from build123d import *

# Parameters (mm, degrees)
F0_W           = 101.6
F0_H           = 50.8
F1_DEPTH       = 101.6
F3_D           = 5.5
F3_CBORE_D     = 9.75
F3_CBORE_DEPTH = 5
F4_R           = 12.7
F5_W           = 38.1
F5_H           = 63.5
F6_DEPTH       = 25.4
F7_R           = 12.7
F8_SIZE        = 6.35


with BuildPart() as f1:
    # F0 (on Top) → F1 (new body, symmetric)
    with BuildSketch(Plane.XY):
        Rectangle(F0_W, F0_H)
    extrude(amount=F1_DEPTH, both=True)

    # F3 (through all)
    with Locations(Plane.XZ.offset(25.4)):
        with Locations((-9.4546508044, 80.2069678903), (23.0063218623, 55.3097166121), (-16.0729084164, -29.151847586), (22.0608543605, -34.1943278909)):
            CounterBoreHole(F3_D / 2, F3_CBORE_D / 2, F3_CBORE_DEPTH)

    # F4
    f4_edges = [f1.edges().sort_by_distance(p)[0] for p in [
        (-50.8, 0, 101.6),
        (50.8, 0, 101.6),
        (-50.8, 0, -101.6),
        (50.8, 0, -101.6),
    ]]
    fillet(f4_edges, radius=F4_R)

    # F5 (on face) → F6 (cut)
    with BuildSketch(Plane.XZ.offset(25.4)):
        with Locations((-19.05, 19.05)):
            Rectangle(F5_W, F5_H)
    extrude(amount=-F6_DEPTH, mode=Mode.SUBTRACT)

    # F7
    f7_edges = [f1.edges().sort_by_distance(p)[0] for p in [
        (0, -12.7, 50.8),
        (-38.1, -12.7, 50.8),
        (-38.1, -12.7, -12.7),
        (0, -12.7, -12.7),
    ]]
    fillet(f7_edges, radius=F7_R)

    # F8
    f8_edges = [f1.edges().sort_by_distance(p)[0] for p in [
        (-34.380256, -25.4, 47.080256),
    ]]
    chamfer(f8_edges, length=F8_SIZE)


solid = f1.part
The model under review builds one solid part; all positions refer to its coordinate system, in mm. A direction names the side the tool comes from. Round coordinates to 2 decimals unless told otherwise and drop trailing zeros. One line per question, with ' | ' between items. Start each with the question number.
Item 1: For pin 1 (7 mm diameter, centred on x = 23.01, z = 55.31, fed in from -Y); pin 2 (3 mm diameter, centred on x = -15.5, z = -28.5, fed in from -Y); pin 3 (11.5 mm diameter, centred on x = -19.5, z = 23, fed in from -Y), all flat-tipped, find the tip position at first contact; note any pin that passes through.
Item 2: Wall thickness on line 1 along X through (y, z) = (-5, 5.5); line 2 along X through (y, z) = (-1, -33.5); line 3 along Z through (x, y) = (-11, -9): over which ranges is each line inside the solid? List them lowest first. Write a range as [from, to].
Item 3: Machinability: for faces 1 (the face through (-41.23, -22.18, 19.32)), 2 (the face through (-47.18, 0.36, 97.78)), which of the approach directions +Z, -Z, +X, -X, +Y, -Y give a long, thin tool a straight path to every point of the face, cutting with its end or side? Answer none if there is none.
Item 4: Draft analysis for pull direction X (two halves, no side actions). For faces 3 (the face through (-1, 0, -101.6)), 4 (the face through (-50.8, 0, 1)), 5 (the face through (-15.715, 2.821, -26.425)), state which applies: +X half, -X half, draft (parallel to the pull), parting line (faces both ways), or undercut.
Return value:
1) pin 1: stops at y = -20.4 | pin 2: passes through | pin 3: stops at y = 0
2) line 1: x = [-50.8, -38.1], [0, 50.8] | line 2: x = [-50.8, 19.4], [24.72, 50.8] | line 3: z = [-101.6, -12.59], [50.69, 77.93], [82.48, 101.6]
3) face 1: -Y | face 2: +Z, -X, +Y, -Y
4) face 3: draft | face 4: -X half | face 5: undercut
